Geometry check sheet. Reference: the model listing, model coordinates, mm. Face numbers are marked on the shaded views. A direction names the side the tool comes from. Coordinates: 2 decimals unless noted, no trailing zeros. Order: outer loops, then holes, each group sorted by start corner. A loop starts at its lowest first (then second) coordinate and runs counter-clockwise, first axis right, second up. Notation, with made-up numbers: (71, 31) - (88, 31) arc R21 ccw to (88, 40) - close; hole circle Ø6 at (33.5, 81.25). An arc over 180 degrees is marked (long way). Put each result on its own line as item: value.
from build123d import *

# Parameters (mm, degrees)
SKETCH1_R                                      = 44
SKETCH1_R_2                                    = 22.5
BOSS_EXTRUDE1_DEPTH                            = 6
CBORE_START                                    = -6
CBORE_SLOT_FOR_M8_HEX_SOCKET_HEAD_CAP_SC_DEPTH = 8.6
CBORE_START_2                                  = 2.6
CBORE_SLOT_FOR_M8_HEX_SOCKET_HEAD_CA_3_DEPTH   = 3.4


with BuildPart() as part:
    # Sketch1 → Boss-Extrude1 (new, symmetric)
    with BuildSketch(Plane.XY):
        Circle(SKETCH1_R)
        Circle(SKETCH1_R_2, mode=Mode.SUBTRACT)
    extrude(amount=BOSS_EXTRUDE1_DEPTH, both=True)

    # CBORE SLOT for M8 Hex Socket Head Cap Screw1: read off the stored shape, not the designer's step
    # CBORE SLOT for M8 Hex Socket Head Ca 2 → CBORE SLOT for M8 Hex Socket Head Cap Screw1 (cut)
    with BuildSketch(Plane.XY.offset(CBORE_START)):
        with BuildLine():
            ThreePointArc((38.439558263, 18.130729877), (28.479840149, 21.778196819), (24.832373207, 11.818478705))
            Line((24.832373207, 11.818478705), (25.04278158, 11.36490587))
            ThreePointArc((25.04278158, 11.36490587), (35.002499693, 7.717438928), (38.649966636, 17.677157041))
            Line((38.649966636, 17.677157041), (38.439558263, 18.130729877))
        make_face()
        with BuildLine():
            ThreePointArc((21.446206215, -28.358257918), (11.486488101, -24.710790976), (7.839021159, -34.67050909))
            Line((7.839021159, -34.67050909), (8.049429531, -35.124081925))
            ThreePointArc((8.049429531, -35.124081925), (18.009147645, -38.771548867), (21.656614587, -28.811830753))
            Line((21.656614587, -28.811830753), (21.446206215, -28.358257918))
        make_face()
        with BuildLine():
            ThreePointArc((-25.04278158, -11.36490587), (-35.002499693, -7.717438928), (-38.649966636, -17.677157041))
            Line((-38.649966636, -17.677157041), (-38.439558263, -18.130729877))
            ThreePointArc((-38.439558263, -18.130729877), (-28.479840149, -21.778196819), (-24.832373207, -11.818478705))
            Line((-24.832373207, -11.818478705), (-25.04278158, -11.36490587))
        make_face()
        with BuildLine():
            ThreePointArc((-8.049429531, 35.124081925), (-18.009147645, 38.771548867), (-21.656614587, 28.811830753))
            Line((-21.656614587, 28.811830753), (-21.446206215, 28.358257918))
            ThreePointArc((-21.446206215, 28.358257918), (-11.486488101, 24.710790976), (-7.839021159, 34.67050909))
            Line((-7.839021159, 34.67050909), (-8.049429531, 35.124081925))
        make_face()
    extrude(amount=CBORE_SLOT_FOR_M8_HEX_SOCKET_HEAD_CAP_SC_DEPTH, mode=Mode.SUBTRACT)

    # CBORE SLOT for M8 Hex Socket Head Ca 3 o → CBORE SLOT for M8 Hex Socket Head Ca 3 (cut)
    with BuildSketch(Plane.XY.offset(CBORE_START_2)):
        with BuildLine():
            ThreePointArc((35.718121252, 16.868279642), (29.742290383, 19.056759808), (27.553810218, 13.080928939))
            Line((27.553810218, 13.080928939), (27.764218591, 12.627356104))
            ThreePointArc((27.764218591, 12.627356104), (33.740049459, 10.438875939), (35.928529624, 16.414706807))
            Line((35.928529624, 16.414706807), (35.718121252, 16.868279642))
        make_face()
        with BuildLine():
            ThreePointArc((18.724769204, -29.620708152), (12.748938336, -27.432227987), (10.56045817, -33.408058855))
            Line((10.56045817, -33.408058855), (10.770866543, -33.86163169))
            ThreePointArc((10.770866543, -33.86163169), (16.746697411, -36.050111856), (18.935177576, -30.074280987))
            Line((18.935177576, -30.074280987), (18.724769204, -29.620708152))
        make_face()
        with BuildLine():
            ThreePointArc((-27.764218591, -12.627356104), (-33.740049459, -10.438875939), (-35.928529624, -16.414706807))
            Line((-35.928529624, -16.414706807), (-35.718121252, -16.868279642))
            ThreePointArc((-35.718121252, -16.868279642), (-29.742290383, -19.056759808), (-27.553810218, -13.080928939))
            Line((-27.553810218, -13.080928939), (-27.764218591, -12.627356104))
        make_face()
        with BuildLine():
            ThreePointArc((-10.770866543, 33.86163169), (-16.746697411, 36.050111856), (-18.935177576, 30.074280987))
            Line((-18.935177576, 30.074280987), (-18.724769204, 29.620708152))
            ThreePointArc((-18.724769204, 29.620708152), (-12.748938336, 27.432227987), (-10.56045817, 33.408058855))
            Line((-10.56045817, 33.408058855), (-10.770866543, 33.86163169))
        make_face()
    extrude(amount=CBORE_SLOT_FOR_M8_HEX_SOCKET_HEAD_CA_3_DEPTH, mode=Mode.SUBTRACT)

    # CBORE SLOT for M8 Hex Socket Head Ca 4: loft between two sections, ruled curve by curve
    cbore_slot_for_m8_hex_socket_head_ca_4_from = [
        Edge.make_three_point_arc((24.832373207, 11.818478705, -5.975), (24.593381518, 17.5537529, -5.975), (28.479840149, 21.778196819, -5.975)),
        Edge.make_three_point_arc((28.479840149, 21.778196819, -5.975), (34.215114344, 22.017188508, -5.975), (38.439558263, 18.130729877, -5.975)),
        Edge.make_three_point_arc((38.649966636, 17.677157041, -5.975), (38.888958324, 11.941882847, -5.975), (35.002499693, 7.717438928, -5.975)),
        Edge.make_three_point_arc((35.002499693, 7.717438928, -5.975), (29.267225499, 7.478447239, -5.975), (25.04278158, 11.36490587, -5.975)),
        Edge.make_line((38.439558263, 18.130729877, -5.975), (38.649966636, 17.677157041, -5.975)),
        Edge.make_line((24.832373207, 11.818478705, -5.975), (25.04278158, 11.36490587, -5.975)),
    ]
    cbore_slot_for_m8_hex_socket_head_ca_4_to = [
        Edge.make_three_point_arc((24.809694565, 11.807958286, -6), (24.569906238, 17.562350062, -6), (28.469319731, 21.800875461, -6)),
        Edge.make_three_point_arc((28.469319731, 21.800875461, -6), (34.223711506, 22.040663789, -6), (38.462236905, 18.141250295, -6)),
        Edge.make_three_point_arc((38.672645277, 17.68767746, -6), (38.912433605, 11.933285685, -6), (35.013020112, 7.694760286, -6)),
        Edge.make_three_point_arc((35.013020112, 7.694760286, -6), (29.258628337, 7.454971958, -6), (25.020102938, 11.354385451, -6)),
        Edge.make_line((38.462236905, 18.141250295, -6), (38.672645277, 17.68767746, -6)),
        Edge.make_line((24.809694565, 11.807958286, -6), (25.020102938, 11.354385451, -6)),
    ]
    cbore_slot_for_m8_hex_socket_head_ca_4 = Solid(Shell([*[Face.make_surface_from_curves(cbore_slot_for_m8_hex_socket_head_ca_4_from[k], cbore_slot_for_m8_hex_socket_head_ca_4_to[k]) for k in range(6)], Face(Wire(cbore_slot_for_m8_hex_socket_head_ca_4_from)), Face(Wire(cbore_slot_for_m8_hex_socket_head_ca_4_to))]))
    add(cbore_slot_for_m8_hex_socket_head_ca_4, mode=Mode.SUBTRACT)

    # CBORE SLOT for M8 Hex Socket Head Ca 5: loft between two sections, ruled curve by curve
    cbore_slot_for_m8_hex_socket_head_ca_5_from = [
        Edge.make_three_point_arc((7.839021159, -34.67050909, -5.975), (7.60002947, -28.935234895, -5.975), (11.486488101, -24.710790976, -5.975)),
        Edge.make_three_point_arc((11.486488101, -24.710790976, -5.975), (17.221762296, -24.471799287, -5.975), (21.446206215, -28.358257918, -5.975)),
        Edge.make_three_point_arc((21.656614587, -28.811830753, -5.975), (21.895606276, -34.547104948, -5.975), (18.009147645, -38.771548867, -5.975)),
        Edge.make_three_point_arc((18.009147645, -38.771548867, -5.975), (12.27387345, -39.010540556, -5.975), (8.049429531, -35.124081925, -5.975)),
        Edge.make_line((21.446206215, -28.358257918, -5.975), (21.656614587, -28.811830753, -5.975)),
        Edge.make_line((7.839021159, -34.67050909, -5.975), (8.049429531, -35.124081925, -5.975)),
    ]
    cbore_slot_for_m8_hex_socket_head_ca_5_to = [
        Edge.make_three_point_arc((7.816342517, -34.681029508, -6), (7.576554189, -28.926637733, -6), (11.475967683, -24.688112334, -6)),
        Edge.make_three_point_arc((11.475967683, -24.688112334, -6), (17.230359458, -24.448324006, -6), (21.468884857, -28.347737499, -6)),
        Edge.make_three_point_arc((21.679293229, -28.801310335, -6), (21.919081557, -34.55570211, -6), (18.019668064, -38.794227509, -6)),
        Edge.make_three_point_arc((18.019668064, -38.794227509, -6), (12.265276288, -39.034015837, -6), (8.02675089, -35.134602343, -6)),
        Edge.make_line((21.468884857, -28.347737499, -6), (21.679293229, -28.801310335, -6)),
        Edge.make_line((7.816342517, -34.681029508, -6), (8.02675089, -35.134602343, -6)),
    ]
    cbore_slot_for_m8_hex_socket_head_ca_5 = Solid(Shell([*[Face.make_surface_from_curves(cbore_slot_for_m8_hex_socket_head_ca_5_from[k], cbore_slot_for_m8_hex_socket_head_ca_5_to[k]) for k in range(6)], Face(Wire(cbore_slot_for_m8_hex_socket_head_ca_5_from)), Face(Wire(cbore_slot_for_m8_hex_socket_head_ca_5_to))]))
    add(cbore_slot_for_m8_hex_socket_head_ca_5, mode=Mode.SUBTRACT)

    # CBORE SLOT for M8 Hex Socket Head Ca 6: loft between two sections, ruled curve by curve
    cbore_slot_for_m8_hex_socket_head_ca_6_from = [
        Edge.make_three_point_arc((-38.649966636, -17.677157041, -5.975), (-38.888958324, -11.941882847, -5.975), (-35.002499693, -7.717438928, -5.975)),
        Edge.make_three_point_arc((-35.002499693, -7.717438928, -5.975), (-29.267225499, -7.478447239, -5.975), (-25.04278158, -11.36490587, -5.975)),
        Edge.make_three_point_arc((-24.832373207, -11.818478705, -5.975), (-24.593381518, -17.5537529, -5.975), (-28.479840149, -21.778196819, -5.975)),
        Edge.make_three_point_arc((-28.479840149, -21.778196819, -5.975), (-34.215114344, -22.017188508, -5.975), (-38.439558263, -18.130729877, -5.975)),
        Edge.make_line((-25.04278158, -11.36490587, -5.975), (-24.832373207, -11.818478705, -5.975)),
        Edge.make_line((-38.649966636, -17.677157041, -5.975), (-38.439558263, -18.130729877, -5.975)),
    ]
    cbore_slot_for_m8_hex_socket_head_ca_6_to = [
        Edge.make_three_point_arc((-38.672645277, -17.68767746, -6), (-38.912433605, -11.933285685, -6), (-35.013020112, -7.694760286, -6)),
        Edge.make_three_point_arc((-35.013020112, -7.694760286, -6), (-29.258628337, -7.454971958, -6), (-25.020102938, -11.354385451, -6)),
        Edge.make_three_point_arc((-24.809694565, -11.807958286, -6), (-24.569906238, -17.562350062, -6), (-28.469319731, -21.800875461, -6)),
        Edge.make_three_point_arc((-28.469319731, -21.800875461, -6), (-34.223711506, -22.040663789, -6), (-38.462236905, -18.141250295, -6)),
        Edge.make_line((-25.020102938, -11.354385451, -6), (-24.809694565, -11.807958286, -6)),
        Edge.make_line((-38.672645277, -17.68767746, -6), (-38.462236905, -18.141250295, -6)),
    ]
    cbore_slot_for_m8_hex_socket_head_ca_6 = Solid(Shell([*[Face.make_surface_from_curves(cbore_slot_for_m8_hex_socket_head_ca_6_from[k], cbore_slot_for_m8_hex_socket_head_ca_6_to[k]) for k in range(6)], Face(Wire(cbore_slot_for_m8_hex_socket_head_ca_6_from)), Face(Wire(cbore_slot_for_m8_hex_socket_head_ca_6_to))]))
    add(cbore_slot_for_m8_hex_socket_head_ca_6, mode=Mode.SUBTRACT)

    # CBORE SLOT for M8 Hex Socket Head Ca 7: loft between two sections, ruled curve by curve
    cbore_slot_for_m8_hex_socket_head_ca_7_from = [
        Edge.make_three_point_arc((-21.656614587, 28.811830753, -5.975), (-21.895606276, 34.547104948, -5.975), (-18.009147645, 38.771548867, -5.975)),
        Edge.make_three_point_arc((-18.009147645, 38.771548867, -5.975), (-12.27387345, 39.010540556, -5.975), (-8.049429531, 35.124081925, -5.975)),
        Edge.make_three_point_arc((-7.839021159, 34.67050909, -5.975), (-7.60002947, 28.935234895, -5.975), (-11.486488101, 24.710790976, -5.975)),
        Edge.make_three_point_arc((-11.486488101, 24.710790976, -5.975), (-17.221762296, 24.471799287, -5.975), (-21.446206215, 28.358257918, -5.975)),
        Edge.make_line((-8.049429531, 35.124081925, -5.975), (-7.839021159, 34.67050909, -5.975)),
        Edge.make_line((-21.656614587, 28.811830753, -5.975), (-21.446206215, 28.358257918, -5.975)),
    ]
    cbore_slot_for_m8_hex_socket_head_ca_7_to = [
        Edge.make_three_point_arc((-21.679293229, 28.801310335, -6), (-21.919081557, 34.55570211, -6), (-18.019668064, 38.794227509, -6)),
        Edge.make_three_point_arc((-18.019668064, 38.794227509, -6), (-12.265276288, 39.034015837, -6), (-8.02675089, 35.134602343, -6)),
        Edge.make_three_point_arc((-7.816342517, 34.681029508, -6), (-7.576554189, 28.926637733, -6), (-11.475967683, 24.688112334, -6)),
        Edge.make_three_point_arc((-11.475967683, 24.688112334, -6), (-17.230359458, 24.448324006, -6), (-21.468884857, 28.347737499, -6)),
        Edge.make_line((-8.02675089, 35.134602343, -6), (-7.816342517, 34.681029508, -6)),
        Edge.make_line((-21.679293229, 28.801310335, -6), (-21.468884857, 28.347737499, -6)),
    ]
    cbore_slot_for_m8_hex_socket_head_ca_7 = Solid(Shell([*[Face.make_surface_from_curves(cbore_slot_for_m8_hex_socket_head_ca_7_from[k], cbore_slot_for_m8_hex_socket_head_ca_7_to[k]) for k in range(6)], Face(Wire(cbore_slot_for_m8_hex_socket_head_ca_7_from)), Face(Wire(cbore_slot_for_m8_hex_socket_head_ca_7_to))]))
    add(cbore_slot_for_m8_hex_socket_head_ca_7, mode=Mode.SUBTRACT)


solid = part.part
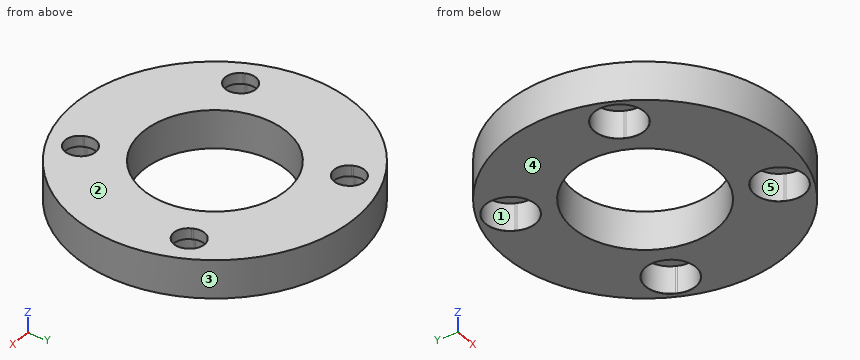
Q1. Section check A-A on y = 0. Record the boundary of the cut face in (x, z), then the cut area to 3 significant figures.
Answer block:
outline: (-44, -6) - (-22.5, -6) - (-22.5, 6) - (-44, 6) - close; (22.5, -6) - (44, -6) - (44, 6) - (22.5, 6) - close
area: 516 mm^2
Q2. Depth check by flat-ended pin: pin 1 Ø4.5 at (x, y) = (14.5, -34.5) entering from -Z; pin 2 Ø2 at (x, z) = (-22.5, 1) entering from -Y; pin 3 Ø6 at (x, z) = (31, -2) entering from -Y. Enter the tip coordinate at first touch or a pass-through.
Answer block:
pin 1: stops at z = 2.6
pin 2: stops at y = -38.39
pin 3: stops at y = -33.94
Q3. Section check D-D on x = 16. State how many separate pieces and enclosed holes the cut face has, then the cut area to 3 significant figures.
Answer block:
separate pieces: 3
enclosed holes: 0
area: 442 mm^2
Q4. Access from +Z, -Z, +X, -X, +Y, -Y to the whole of each face (thin tool, end or side, straight path). Record for the marked faces 1 and 2.
Answer block:
face 1: -Z
face 2: +Z, +X, -X, +Y, -Y
Q5. Draft check along Y on the marked faces 3, 4 and 5. Enter one of: pulls with the +Y half, pulls with the -Y half, needs draft (parallel to the pull), parting line crosses it, or undercut.
Answer block:
face 3: parting line crosses it
face 4: needs draft
face 5: undercut
Q6. Section check C-C on z = 1. Record the boundary of the cut face in (x, y), then the cut area to 3 significant figures.
Answer block:
outline: circle Ø88 at (0, 0); hole (-38.65, -17.68) - (-38.44, -18.13) arc R7.5 ccw to (-24.83, -11.82) - (-25.04, -11.36) arc R7.5 ccw to start; hole circle Ø45 at (0, 0); hole (-21.66, 28.81) - (-21.45, 28.36) arc R7.5 ccw to (-7.84, 34.67) - (-8.05, 35.12) arc R7.5 ccw to start; hole (7.84, -34.67) - (8.05, -35.12) arc R7.5 ccw to (21.66, -28.81) - (21.45, -28.36) arc R7.5 ccw to start; hole (24.83, 11.82) - (25.04, 11.36) arc R7.5 ccw to (38.65, 17.68) - (38.44, 18.13) arc R7.5 ccw to start
area: 3,750 mm^2
Q7. Thickness scan on L1, parallel to Y at x = 0, z = -1.25; L2, parallel to Y at x = -13.5, z = -4; L3, parallel to Y at x = 11, z = 0. Record the ranges inside material, lowest first. Write a range as [from, to].
Answer block:
L1: y = [-44, -22.5], [22.5, 44]
L2: y = [-41.88, -18], [18, 24.1], [39.34, 41.88]
L3: y = [-42.6, -38.4], [-24.96, -19.63], [19.63, 42.6]
